Autodesk Inventor part; units mm, degrees
ref_plane "YZ Plane" through (0, 0, 0) normal (1, 0, 0) x (0, 1, 0)
ref_plane "XZ Plane" through (0, 0, 0) normal (0, 1, 0) x (-1, 0, 0)
ref_plane "XY Plane" through (0, 0, 0) normal (0, 0, 1) x (1, 0, 0)
sketch "Sketch1" plane through (0, 0, 0) normal (0, 1, 0) x (-1, 0, 0)
  line L0 (0, 0) -> (0, -145)
  line L1 (0, -145) -> (3, -145)
  line L2 (3, -145) -> (8, -145)
  circle A0 centre (8, -145) radius 1.5
  line L3 (0, 0) -> (40, 0)
  line L4 (0, -145) -> (0, -250)
  line L5 (0, -250) -> (8, -250)
  line L6 (8, -156) -> (8, -148)
  circle A1 centre (8, -145) radius 3
  line L7 (13, -250) -> (8, -250)
  line L8 (8, -156) -> (13, -156)
  line L9 (13, -156) -> (13, -166)
  line L10 (10.3705, -134.2585) -> (15.1383, -135.3107)
  line L11 (15.1383, -135.3107) -> (14.892, -136.4268)
  line L12 (15.1383, -135.3107) -> (17.2934, -125.5456)
  line L13 (17.2934, -125.5456) -> (12.5256, -124.4934)
  line L14 (17.2934, -125.5456) -> (22.1759, -126.6232)
  line L15 (13, -166) -> (18, -166)
  line L16 (22.1759, -126.6232) -> (22.1759, -166)
  line L17 (22.1759, -166) -> (18, -166)
  arc A2 (0, -137.4502) -> (0, -152.5498) centre (8, -145) ccw
  arc A3 (8, -156) -> (10.3705, -134.2585) centre (8, -145) ccw
  line L18 (40, 0) -> (12.5256, -124.4934)
  line L19 (10.3705, -134.2585) -> (8.6465, -142.0705)
  line L20 (8, -148) -> (8, -153)
  arc A4 (0, -142.1277) -> (0, -147.8723) centre (8, -145) ccw
  arc A5 (8, -153.5) -> (9.8318, -136.6997) centre (8, -145) ccw
  line L21 (8, -153.5) -> (8, -156)
  line L22 (9.8318, -136.6997) -> (10.3705, -134.2585)
  line L23 (9.5, -145) -> (11.2347, -137.1396)
  line L24 (9.5, -145) -> (16.5, -145)
  line L25 (13, -156) -> (13, -154.798)
  line L26 (16.5, -145) -> (19, -145)
  line L27 (11.2347, -137.1396) -> (11.7798, -134.6698)
  dimension "d4" = 3
  dimension "d0" = 145
  dimension "d1" = 3
  dimension "d2" = 5
  dimension "d5" = 40
  dimension "d6" = 105
  dimension "d8" = 6
  dimension "d10" = 10
  dimension "d11" = 10
  dimension "d12" = 5
  dimension "d13" = 5
extrude "Extrusion4" add sketch "Sketch1" along normal mid plane 28 contours L14 L16 L17 L15 L9 L25 A3 L11 L12 | A1 L23 A0 L2 | L2 A0 L24 A1 | A3 L27 A5 L19 | A3 L26 A5 L27 | L19 A5 L23 A1 | A1 L24 A5 L6 | A3 L6 A5 L26 | L23 A1 L24 | L23 A5 L24 A1
extrude "Extrusion5" cut sketch "Sketch1" along normal mid plane 18.5 contours A1 L23 A0 L2 | L2 A0 L24 A1 | L19 A5 L23 A1 | A1 L24 A5 L6 | L23 A1 L24 | L23 A5 L24 A1
extrude "Extrusion6" cut sketch "Sketch1" along normal mid plane 10.5 contours A3 L27 A5 L19 | A3 L26 A5 L27 | A3 L6 A5 L26
extrude "Extrusion7" add sketch "Sketch1" along normal mid plane 9.5 contours A3 L26 A5 L27 | L23 A1 L24 | L23 A5 L24 A1
sketch "Sketch2" plane through (-17.2934, -14, -125.5456) normal (0.9765029, 0, 0.2155041) x (0.2155041, 0, -0.9765029)
  line L0 (0, 28) -> (0, 14)
  line L1 (0, 0) -> (0, 28)
  line L2 (0, 14) -> (5, 14)
  line L3 (5, 14) -> (5, 21)
  line L4 (5, 14) -> (5, 7)
  circle A0 centre (5, 21) radius 2.4
  circle A1 centre (5, 7) radius 2.4
  circle A2 centre (5, 21) radius 4
  circle A3 centre (5, 7) radius 4
  point P0 (-118.8689, 14)
  dimension "d29" = 5
  dimension "d30" = 7
  dimension "d31" = 7
  dimension "d32" = 4.8
  dimension "d33" = 4.8
  dimension "d34" = 8
  dimension "d35" = 8
extrude "Extrusion8" cut sketch "Sketch2" against normal blind 10.5 contours A0 | A1 | A2 | A3
extrude "Extrusion9" add sketch "Sketch2" against normal blind 5
sketch "Sketch3" plane through (-13, -14, -166) normal (1, 0, 0) x (0, 0, -1)
  line L0 (0, 28) -> (0, 14)
  line L1 (0, 0) -> (0, 28)
  line L2 (0, 14) -> (-5, 14)
  line L3 (-5, 14) -> (-5, 21)
  line L4 (-5, 14) -> (-5, 7)
  circle A0 centre (-5, 21) radius 2.4
  circle A1 centre (-5, 7) radius 2.4
  point P0 (-166, 14)
  dimension "d40" = 5
  dimension "d41" = 7
  dimension "d42" = 7
  dimension "d43" = 4.8
  dimension "d44" = 4.8
extrude "Extrusion10" cut sketch "Sketch3" against normal blind 10
properties part number "push_clip"
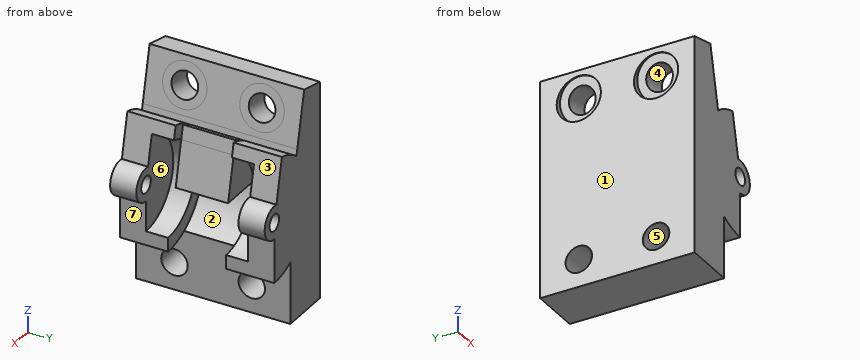
Work out the finished part from the listing and answer in its coordinate system (mm). Face numbers are marked on the shaded views. A direction names the side the tool comes from. Give positions to 0.01 mm unless a question says otherwise; leave off trailing zeros. Loops run counter-clockwise (first coordinate to the right, second up) from the corner with the lowest first, then second, coordinate; pieces in that order, holes last. Notation, with made-up numbers: (5.5, 19) -> (21.5, 19) arc R15 cw to (21.5, 25) -> close; hole circle Ø7 at (-6.75, -3). An arc over 180 degrees is marked (long way). Use a Markdown table: item, result. Add a question column.
1. Section C-C on x = -14.25 is taken. Determine the outline of the cut face in (y, z).
2. Find the intervals of material crossed by probe 1 along Y at (x, z) = (-18.75, -161); probe 2 along Y at (x, z) = (-11.75, -145.5); probe 3 along Z at (x, y) = (-19, -7), in increasing order.
3. Flat-ended cylindrical pins translate along their axes: pin 1 Ø9 at (y, z) = (5.5, -159) entering from +X; pin 2 Ø4 at (y, z) = (7, -161) entering from +X. Find the tip coordinate at first contact, or state that the pin passes through.
4. For the marked faces 5, 6 and 7, determine the directions among +Z, -Z, +X, -X, +Y, -Y from which every point of the face is accessible in a straight line to the end or side of a thin tool.
5. Section D-D on y = 7 is taken. Determine the outline of the cut face in (x, z).
6. Section A-A on y = -2.5 is taken. Determine the outline of the cut face in (x, z), and give its area (3 significant figures).
7. Determine the mould class of the marked faces 1, 2, 3 and 4 for opening direction Z: released by +Z, released by -Z, zero draft, split by the parting line, or undercut.
8. Section B-B on z = -161 is taken. Determine the outline of the cut face in (x, y).
Results below:
| question | item | result |
|---|---|---|
| 1 | outline | (-14, -166) -> (14, -166) -> (14, -135.95) -> (5.25, -135.95) -> (5.25, -139.24) -> (9.25, -139.24) -> (9.25, -150.76) -> (5.25, -150.76) -> (5.25, -154.05) -> (-5.25, -154.05) -> (-5.25, -150.76) -> (-9.25, -150.76) -> (-9.25, -139.24) -> (-5.25, -139.24) -> (-5.25, -135.95) -> (-14, -135.95) -> close; (-4.75, -145) -> (4.75, -145) -> (4.75, -135.95) -> (-4.75, -135.95) -> close; hole circle Ø4.8 at (-7, -161); hole circle Ø4.8 at (7, -161) |
| 2 | probe 1 | y = -14 to -9.4, -4.6 to 4.6, 9.4 to 14 |
| 2 | probe 2 | y = -14 to -9.25, 9.25 to 14 |
| 2 | probe 3 | z = -166 to -163.4, -158.6 to -133.5, -128.58 to -125.92 |
| 3 | pin 1 | stops at x = -8 |
| 3 | pin 2 | passes through |
| 4 | face 5 | +X, -X |
| 4 | face 6 | +X |
| 4 | face 7 | -Z, +X, +Y, -Y |
| 5 | outline | (-22.18, -166) -> (-13, -166) -> (-13, -163.4) -> (-22.18, -163.4) -> close; (-22.18, -158.6) -> (-13, -158.6) -> (-13, -154.8) arc R11 ccw to (-8, -156) -> (-8, -153.5) arc R8.5 cw to (-9.83, -136.7) -> (-10.37, -134.26) arc R11 ccw to (-14.89, -136.43) -> (-15.14, -135.31) -> (-15.35, -134.33) -> (-15.7, -132.77) -> (-20.58, -133.85) -> (-20.24, -135.41) -> (-22.18, -135.84) -> close; (-22.18, -127.65) -> (-21.96, -127.6) -> (-21.62, -129.16) -> (-16.73, -128.08) -> (-17.08, -126.52) -> (-17.29, -125.55) -> (-22.18, -126.62) -> close |
| 6 | outline | (-22.18, -166) -> (-13, -166) -> (-13, -154.8) arc R11 cw to (-19, -145) -> (-9.5, -145) -> (-11.23, -137.14) -> (-11.78, -134.67) arc R11 ccw to (-14.89, -136.43) -> (-15.14, -135.31) -> (-17.29, -125.55) -> (-22.18, -126.62) -> close |
| 6 | area | 318 mm^2 |
| 7 | face 1 | zero draft |
| 7 | face 2 | undercut |
| 7 | face 3 | released by +Z |
| 7 | face 4 | undercut |
| 8 | outline | (-22.18, -14) -> (-13, -14) -> (-13, -9.4) -> (-22.18, -9.4) -> close; (-22.18, -4.6) -> (-13, -4.6) -> (-13, 4.6) -> (-22.18, 4.6) -> close; (-22.18, 9.4) -> (-13, 9.4) -> (-13, 14) -> (-22.18, 14) -> close |
